Part model, mm, in its own coordinate system. Round coordinates to 2 decimals unless told otherwise and drop trailing zeros. Loops run counter-clockwise (first coordinate to the right, second up) from the corner with the lowest first, then second, coordinate; pieces in that order, holes last.
1) Band-saw the part on A-A, the plane y = -7.5. Write the cut outline in (x, z), then the cut area to 3 significant figures.
2) Drop flat-ended pins along their axis: P1, Ø10, axis at y = -9.5, z = -23, coming from the +X side; P2, Ø1, axis at y = -17.5, z = -16, coming from the -X side; P3, Ø4, axis at x = -189.5, y = -15.5, coming from the +Z side. Give the stop position or say it passes through.
3) Probe line 1 (Z direction, x = -327.5, y = -14.75); line 2 (X direction, y = -11, z = -2); line 3 (Z direction, x = 0.5, y = -11.5). List the from-to ranges inside material, lowest first.
4) Band-saw the part on B-B, the plane x = 241. Write the cut outline in (y, z), then the cut area to 3 significant figures.
5) Band-saw the part on C-C, the plane z = -36.5. Write the cut outline in (x, y), then the cut area to 3 significant figures.
from build123d import *

# Parameters (mm, degrees)
F1_DEPTH = 20


with BuildPart() as f1:
    # F0 (on Front) → F1 (new body)
    with BuildSketch(Plane.XZ):
        with BuildLine():
            ThreePointArc((-326.583678, 45.472431), (-293.391515, 32.728484), (-279.5, 0))
            Line((-279.5, 0), (279.5, 0))
            ThreePointArc((279.5, 0), (293.168529, 32.511651), (325.961867, 45.489832))
            ThreePointArc((325.961867, 45.489832), (-0.311198, 56.468207), (-326.583678, 45.472431))
        make_face()
        with BuildLine():
            Line((279.5, 0), (-279.5, 0))
            ThreePointArc((-279.5, 0), (-293.933876, -33.243735), (-328.077844, -45.39578))
            ThreePointArc((-328.077844, -45.39578), (0, -56.504902), (328.077844, -45.39578))
            ThreePointArc((328.077844, -45.39578), (293.933876, -33.243735), (279.5, 0))
        make_face()
        with BuildLine():
            ThreePointArc((-328.077844, -45.39578), (-293.933876, -33.243735), (-279.5, 0))
            ThreePointArc((-279.5, 0), (-293.391515, 32.728484), (-326.583678, 45.472431))
            ThreePointArc((-326.583678, 45.472431), (-370.49385, 0.748065), (-328.077844, -45.39578))
        make_face()
        with BuildLine():
            ThreePointArc((325.961867, 45.489832), (293.168529, 32.511651), (279.5, 0))
            ThreePointArc((279.5, 0), (293.933876, -33.243735), (328.077844, -45.39578))
            ThreePointArc((328.077844, -45.39578), (358.243735, -31.066124), (370.5, 0))
            ThreePointArc((370.5, 0), (357.511651, 31.831471), (325.961867, 45.489832))
        make_face()
    extrude(amount=F1_DEPTH)


solid = f1.part
Reported:
1. outline: (-328.08, -45.4) arc R4850 ccw to (328.08, -45.4) arc R45.5 ccw to (325.96, 45.49) arc R4850 ccw to (-326.58, 45.47) arc R45.5 ccw to start
1. area: 75,200 mm2
2. P1: stops at x = 366.79
2. P2: stops at x = -367.78
2. P3: stops at z = 52.85
3. line 1: z = -45.43 to 45.43
3. line 2: x = -370.46 to 370.46
3. line 3: z = -56.5 to 56.47
4. outline: (-20, -50.51) - (0, -50.51) - (0, 50.47) - (-20, 50.47) - close
4. area: 2,020 mm2
5. outline: (-352.17, -20) - (352.17, -20) - (352.17, 0) - (-352.17, 0) - close
5. area: 14,100 mm2
